from build123d import *

# Parameters (mm, degrees)
SKETCH_2_R               = 1.7
CUT_EXTRUDE_1_DEPTH      = 10
CUT_EXTRUDE_2_DEPTH      = 21.273134933
CUT_EXTRUDE_2_DEPTH_BACK = 21.273134933
SKETCH_3_R               = 1.7


with BuildPart() as part:
    # 草图1 → 旋转1 (revolve)
    with BuildSketch(Plane.XY, mode=Mode.PRIVATE) as revolve_1_sk:
        Polygon((-2.5, 0), (-11, 0), (-11, -3), (-5, -3), (-5, -13), (-2.5, -13), align=None)
    revolve(revolve_1_sk.sketch.rotate(Axis((0, 0, 0), (0, -1, 0)), 270), axis=Axis((0, 0, 0), (0, -1, 0)))

    # 草图2 → 切除-拉伸1 (cut)
    with BuildSketch(Plane(origin=(0, 0, 0), x_dir=(1, 0, 0), z_dir=(0, 1, 0))):
        with Locations(Location((0, 8, 0), (0, 0, 270))):
            Circle(SKETCH_2_R)
        with Locations(Location((8, 0, 0), (0, 0, 270))):
            Circle(SKETCH_2_R)
        with Locations(Location((0, -8, 0), (0, 0, 270))):
            Circle(SKETCH_2_R)
        with Locations(Location((-8, 0, 0), (0, 0, 270))):
            Circle(SKETCH_2_R)
    extrude(amount=-CUT_EXTRUDE_1_DEPTH, mode=Mode.SUBTRACT)

    # 草图3 → 切除-拉伸2 (cut, two sides: drawn at the far end of the back side and taken through both)
    with BuildSketch(Plane.XY.offset(-CUT_EXTRUDE_2_DEPTH_BACK)):
        with Locations((0, -8)):
            Circle(SKETCH_3_R)
    extrude(amount=CUT_EXTRUDE_2_DEPTH + CUT_EXTRUDE_2_DEPTH_BACK, mode=Mode.SUBTRACT)


solid = part.part
Input: part model. Units: mm. Frame: model coordinates. Coordinates: 2 decimals unless noted, no trailing zeros. Loops run counter-clockwise (first coordinate to the right, second up) from the corner with the lowest first, then second, coordinate; pieces in that order, holes last. Notation, with made-up numbers: (85, 45.25) -> (97, 45.25) arc R13 ccw to (97, 60.25) -> close; hole circle Ø5 at (1.5, 23). An arc over 180 degrees is marked (long way). Write each question's results on one line, items separated by ' | '. Start each with the question number.
Q1. Section D-D, the plane y = -4.5. Return the cut outline in (x, z).
Q2. Pull-direction query (Z, two-part tool) for faces 1 (the cylindrical face through (-9.66, -1.48, -0.37)), 2 (the cylindrical face through (1.915, -8.07, 4.619)), 3 (the flat face through (5, -3, 2)); classes: released by +Z, released by -Z, zero draft, split by the parting line, or undercut.
Q3. Pin query (flat end, axial travel): pin 1 (2 mm diameter, centred on x = -2.5, y = -9.5, fed in from +Z); pin 2 (5.5 mm diameter, centred on x = 0, y = -8, fed in from +Z); pin 3 (1 mm diameter, centred on x = -4.5, y = -10.5, fed in from -Z). Return the tip coordinate at first contact, or that it passes through.
Q4. Section A-A, the plane z = 0. Return the cut outline in (x, y), plus the area to 3 significant figures.
Q5. Section B-B, the plane x = 0. Return the cut outline in (y, z), plus the area to 3 significant figures.
Q6. Section C-C, the plane x = 7.25. Return the cut outline in (y, z).
Q7. Ray query, line 1 (X direction, y = -2.35, z = 0); line 2 (Y direction, x = 0, z = -3.4); line 3 (X direction, y = -2.5, z = 1.5). Return the intervals inside material, ascending. Write a range as from..to.
Found:
1) outline: circle Ø10 at (0, 0); hole circle Ø5 at (0, 0)
2) face 1: undercut | face 2: split by the parting line | face 3: zero draft
3) pin 1: z = 4.77 | pin 2: z = 5 | pin 3: z = -3
4) outline: (-11, -3) -> (-9.7, -3) -> (-9.7, 0) -> (-11, 0) -> close; (-6.3, -3) -> (-5, -3) -> (-5, -13) -> (-2.5, -13) -> (-2.5, 0) -> (-6.3, 0) -> close; (2.5, -13) -> (5, -13) -> (5, -3) -> (6.3, -3) -> (6.3, 0) -> (2.5, 0) -> close; (9.7, -3) -> (11, -3) -> (11, 0) -> (9.7, 0) -> close | area: 80.6 mm2
5) outline: (-13, -5) -> (-9.7, -5) -> (-9.7, -2.5) -> (-13, -2.5) -> close; (-13, 2.5) -> (-9.7, 2.5) -> (-9.7, 5) -> (-13, 5) -> close; (-6.3, -5) -> (-3, -5) -> (-3, -6.3) -> (0, -6.3) -> (0, -2.5) -> (-6.3, -2.5) -> close; (-6.3, 2.5) -> (0, 2.5) -> (0, 6.3) -> (-3, 6.3) -> (-3, 5) -> (-6.3, 5) -> close; (-3, -11) -> (0, -11) -> (0, -9.7) -> (-3, -9.7) -> close; (-3, 9.7) -> (0, 9.7) -> (0, 11) -> (-3, 11) -> close | area: 63.6 mm2
6) outline: (-3, -8.27) -> (0, -8.27) -> (0, -1.53) -> (-3, -1.53) -> close; (-3, 1.53) -> (0, 1.53) -> (0, 8.27) -> (-3, 8.27) -> close
7) line 1: -11..-9.7, -6.3..-2.5, 2.5..6.3, 9.7..11 | line 2: -13..-9.7, -6.3..0 | line 3: -10.9..-8.8, -7.2..-2, 2..7.2, 8.8..10.9
